Answer from the drawing. Dimensions are ordinates in mm from the lowest x, y and z of the part. A direction names the side the tool comes from. Coordinates: 2 decimals unless noted, no trailing zeros. Order: outer loops, then holes, each group sorted by start corner. A loop starts at its lowest first (then second) coordinate and runs counter-clockwise, first axis right, second up. Notation, with made-up numbers: (-28, 60.25) -> (31, 60.25) arc R17 cw to (31, 89.25) -> close; hole circle Ø4 at (29.25, -7.75). An arc over 180 degrees is marked (long way). Answer as a JSON object with one key per item and string values. Group by question number.
1) Section D-D on z = 0.5 is taken. Determine the outline of the cut face in (x, y).
2) Section B-B on y = 13 is taken. Determine the outline of the cut face in (x, z).
3) Section A-A on x = 7 is taken. Determine the outline of the cut face in (y, z) (1 decimal).
4) A tool of negligible diameter and unlimited length cuts with its end or side. For the marked faces 1, 2, 3, 4 and 5, from which of +Z, -Z, +X, -X, +Y, -Y can it reach the whole face along a straight path? Write none if from no direction.
5) Consider L1, parallel to Z at x = 6.25, y = 17.75; L2, parallel to X at y = 11.75, z = 4.5; L3, parallel to Z at x = 7.25, y = 11.25. Determine where each line is inside the solid, lowest interval first.
6) Section C-C on x = 4 is taken. Determine the outline of the cut face in (y, z).
7) Given pin 1 (3 mm diameter, centred on x = 6.5, z = 4, fed in from +Y); pin 2 (1.5 mm diameter, centred on x = 7.5, z = 5, fed in from -Y); pin 3 (3 mm diameter, centred on x = 3.5, y = 19, fed in from +Z), each flat-ended and moving along its own axis, determine where each tip first touches the part or whether it passes through.
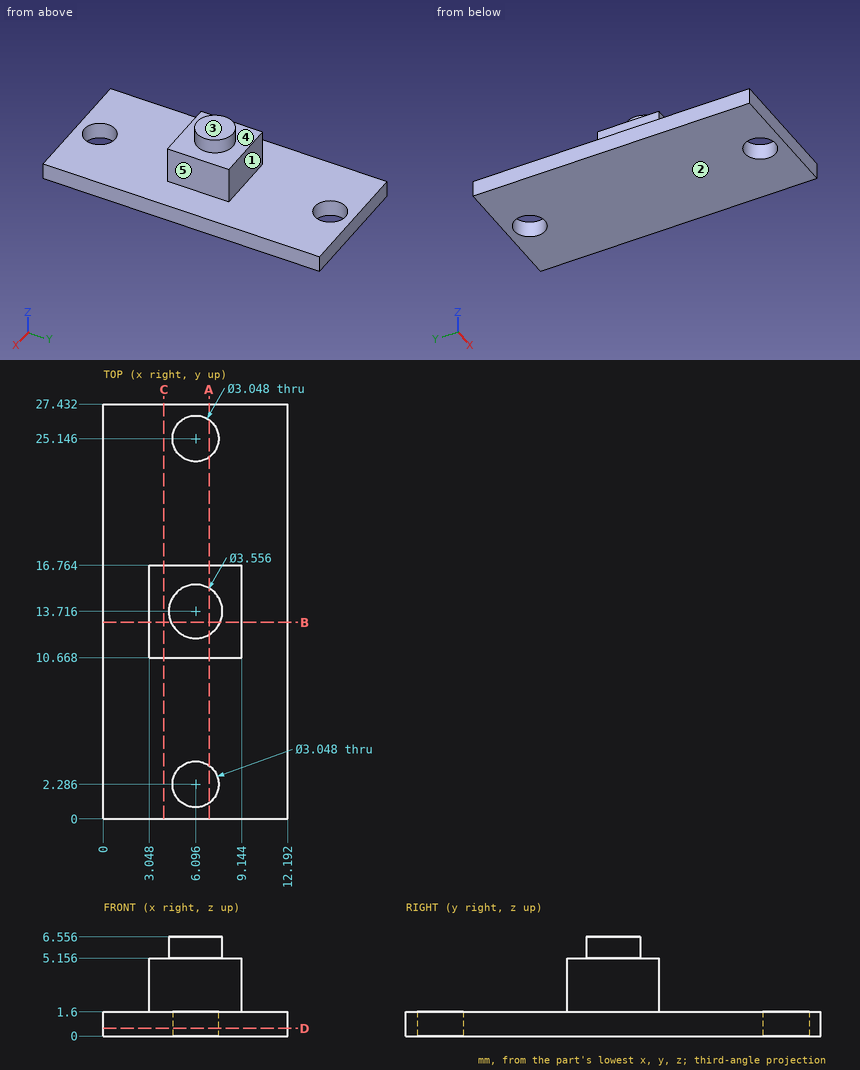
Worked answers:
{
 "1": {"outline": "(0, 0) -> (12.19, 0) -> (12.19, 27.43) -> (0, 27.43) -> close; hole circle Ø3.05 at (6.1, 2.29); hole circle Ø3.05 at (6.1, 25.15)"},
 "2": {"outline": "(0, 0) -> (12.19, 0) -> (12.19, 1.6) -> (9.14, 1.6) -> (9.14, 5.16) -> (7.72, 5.16) -> (7.72, 6.56) -> (4.47, 6.56) -> (4.47, 5.16) -> (3.05, 5.16) -> (3.05, 1.6) -> (0, 1.6) -> close"},
 "3": {"outline": "(0, 0) -> (1.1, 0) -> (1.1, 1.6) -> (0, 1.6) -> close; (3.5, 0) -> (23.9, 0) -> (23.9, 1.6) -> (16.8, 1.6) -> (16.8, 5.2) -> (15.2, 5.2) -> (15.2, 6.6) -> (12.2, 6.6) -> (12.2, 5.2) -> (10.7, 5.2) -> (10.7, 1.6) -> (3.5, 1.6) -> close; (26.4, 0) -> (27.4, 0) -> (27.4, 1.6) -> (26.4, 1.6) -> close"},
 "4": {"face 1": "+Z, +X, -X, +Y", "face 2": "-Z, +X, -X, +Y, -Y", "face 3": "+Z, +X, -X, +Y, -Y", "face 4": "+Z", "face 5": "+Z, +X, +Y, -Y"},
 "5": {"L1": "z = 0 to 1.6", "L2": "x = 3.05 to 9.14", "L3": "z = 0 to 5.16"},
 "6": {"outline": "(0, 0) -> (27.43, 0) -> (27.43, 1.6) -> (16.76, 1.6) -> (16.76, 5.16) -> (10.67, 5.16) -> (10.67, 1.6) -> (0, 1.6) -> close"},
 "7": {"pin 1": "stops at y = 16.76", "pin 2": "stops at y = 10.67", "pin 3": "stops at z = 1.6"}
}
